Check sheet for the modelled part. Datum: model origin and axes. Units: mm. Give positions to 0.01 mm unless a question says otherwise; leave off trailing zeros. Loops run counter-clockwise (first coordinate to the right, second up) from the corner with the lowest first, then second, coordinate; pieces in that order, holes last. Notation, with made-up numbers: (17, 2) - (45, 2) arc R21 cw to (45, 34) - close; hole circle Ø5 at (-19.5, 41.5). An arc over 180 degrees is marked (long way). Answer in a Markdown table with one row per item. Add a question column.
(1) Sectioned sample at B-B on y = 32. Enter the section's corners in (x, z).
(2) Sectioned sample at A-A on z = -24.5. Enter the section's corners in (x, y) (3 decimals), then the cut area to 3 significant figures.
(3) Thickness scan on L1, parallel to X at y = 47.5, z = -24; L2, parallel to X at y = 111, z = -74 (3 decimals). Record the ranges inside material, lowest first.
(4) Sectioned sample at C-C on x = 21. Enter the section's corners in (y, z), then the cut area to 3 significant figures.
(5) Go/stop test with a flat-tipped pin: P1, Ø12, axis at y = 76.5, z = -32, coming from the -X side. Record where the tip stops, or that it passes through.
from build123d import *

# Parameters (mm, degrees)
F0_W     = 31.75
F0_H     = 127
F1_DEPTH = 88.9


with BuildPart() as f1:
    # F0 (on Top) → F1 (new body)
    with BuildSketch(Plane.XY):
        with Locations((0, 63.5)):
            Rectangle(F0_W, F0_H)
        Polygon((-15.875, 0), (-25.4, 0), (-25.4, -133.35), (25.4, -133.35), (25.4, 0), (15.875, 0), align=None)
        Polygon((15.875, 127), (15.875, 0), (25.4, 0), align=None)
        Polygon((-15.875, 127), (-25.4, 0), (-15.875, 0), align=None)
    extrude(amount=-F1_DEPTH)


solid = f1.part
Reply:
| question | item | result |
|---|---|---|
| 1 | outline | (-23, -88.9) - (23, -88.9) - (23, 0) - (-23, 0) - close |
| 2 | outline | (-25.4, -133.35) - (25.4, -133.35) - (25.4, 0) - (15.875, 127) - (-15.875, 127) - (-25.4, 0) - close |
| 2 | area | 12,000 mm^2 |
| 3 | L1 | -21.84 to 21.84 |
| 3 | L2 | -17.075 to 17.075 |
| 4 | outline | (-133.35, -88.9) - (58.67, -88.9) - (58.67, 0) - (-133.35, 0) - close |
| 4 | area | 17,100 mm^2 |
| 5 | P1 | x = -20.11 |
